from build123d import *

# Parameters (mm, degrees)
SKETCH_R  = 1.5
PAD_DEPTH = 3


with BuildPart() as part:
    # Sketch → Pad (new body)
    with BuildSketch(Plane.XY):
        with BuildLine():
            ThreePointArc((-11.777104, -12.530641), (-10.79761, -16.948853), (-6.379399, -15.969359))
            Line((-6.379399, -15.969359), (2.698853, -1.719359))
            ThreePointArc((2.698853, -1.719359), (3.07216, -0.895453), (3.2, 0))
            Line((3.2, 30), (3.2, 0))
            ThreePointArc((3.2, 30), (6.55, 33.35), (3.2, 36.7))
            ThreePointArc((3.2, 36.7), (-1.537615, 34.737615), (-3.5, 30))
            Line((-3.5, 0.461809), (-3.5, 30))
            Line((-11.777104, -12.530641), (-3.5, 0.461809))
        make_face()
        with Locations((-9.078251, -14.25)):
            Circle(SKETCH_R, mode=Mode.SUBTRACT)
        Circle(SKETCH_R, mode=Mode.SUBTRACT)
    extrude(amount=PAD_DEPTH)


solid = part.part
Read the model definition and answer for the solid it produces. Units are mm, in the model's axes. A direction names the side the tool comes from. Round coordinates to 2 decimals unless told otherwise and drop trailing zeros. Loops run counter-clockwise (first coordinate to the right, second up) from the corner with the lowest first, then second, coordinate; pieces in that order, holes last.
Q1. Section B-B on y = -14.25 is taken. Write down the section's boundary in (x, z).
Q2. Section C-C on x = 0 is taken. Write down the section's boundary in (y, z).
Q3. Which of the six approach directions +Z, -Z, +X, -X, +Y, -Y give full straight-line access (tool end or side, diameter ignored) to faces 1 (the face through (-3.5, 15, 1)), 2 (the face through (3.069, -0.908, 1.479))?
Q4. Section D-D on y = 12 is taken. Write down the section's boundary in (x, z).
Q5. Determine the mould class of faces 3 (the face through (-1.9, -8.94, 1.48)), 4 (the face through (-10.577, -14.184, 1.479)), 5 (the face through (-1.5, 0.07, 1.48)), 6 (the face through (3.2, 15, 1)) for opening direction Y: released by +Y, released by -Y, zero draft, split by the parting line, or undercut.
Q6. This flat-tipped pin is pushed along its axis until it touches: pin 1 (1.5 mm diameter, centred on y = -4, z = 1, fed in from +X). Where does it stop, or does it pass through?
Q7. Consider probe 1 along Y at (x, z) = (0.5, 2.65); probe 2 along X at (y, z) = (25.5, 1.4); probe 3 along Y at (x, z) = (0, 2.1). Determine where each line is inside the solid, lowest interval first.
Q8. Section A-A on z = 1.05 is taken. Write down the section's boundary in (x, y), and give its area (3 significant figures).
Output:
1. outline: (-12.28, 0) - (-10.58, 0) - (-10.58, 3) - (-12.28, 3) - close; (-7.58, 0) - (-5.28, 0) - (-5.28, 3) - (-7.58, 3) - close
2. outline: (-5.96, 0) - (-1.5, 0) - (-1.5, 3) - (-5.96, 3) - close; (1.5, 0) - (35.89, 0) - (35.89, 3) - (1.5, 3) - close
3. face 1: +Z, -Z, -X, +Y
3. face 2: +Z, -Z, +X, -Y
4. outline: (-3.5, 0) - (3.2, 0) - (3.2, 3) - (-3.5, 3) - close
5. face 3: released by -Y
5. face 4: undercut
5. face 5: undercut
5. face 6: zero draft
6. pin 1: stops at x = 1.72
7. probe 1: y = -5.17 to -1.41, 1.41 to 36.13
7. probe 2: x = -3.5 to 3.2
7. probe 3: y = -5.96 to -1.5, 1.5 to 35.89
8. outline: (-11.78, -12.53) arc R3.2 ccw to (-6.38, -15.97) - (2.7, -1.72) arc R3.2 ccw to (3.2, 0) - (3.2, 30) arc R3.35 ccw to (3.2, 36.7) arc R6.7 ccw to (-3.5, 30) - (-3.5, 0.46) - close; hole circle Ø3 at (-9.08, -14.25); hole circle Ø3 at (0, 0)
8. area: 364 mm2
